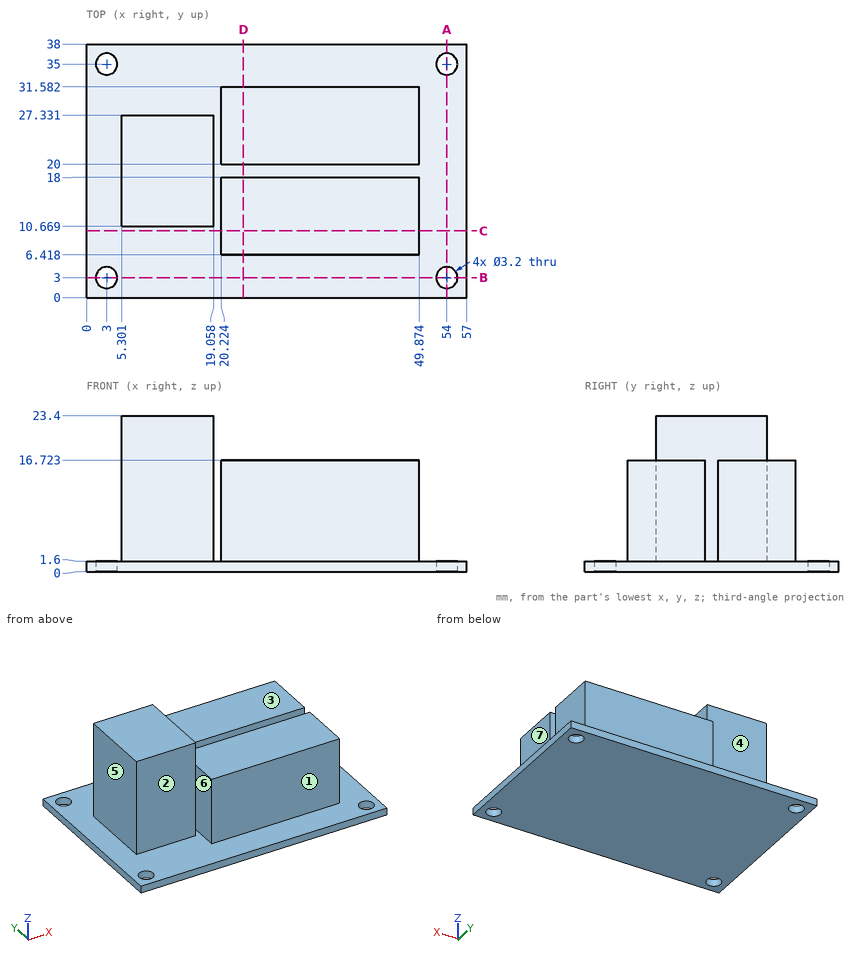
For this review, use the dimensioned drawing (mm, ordinates from the lowest corner) and the shaded views. A direction names the side the tool comes from. Round coordinates to 2 decimals unless told otherwise and drop trailing zeros. Loops run counter-clockwise (first coordinate to the right, second up) from the corner with the lowest first, then second, coordinate; pieces in that order, holes last. Notation, with made-up numbers: M 63,-9 L 111,-9 A22 ccw 111,5 Z; hole C 28,-10.75 d10. An arc over 180 degrees is marked long. Answer as CSV lines item,"result".
1. We need section D-D (x = 23.5). Give the boundary of the cut face in (y, z).
Outcome:
outline,"M 0,0 L 38,0 L 38,1.6 L 31.58,1.6 L 31.58,16.72 L 20,16.72 L 20,1.6 L 18,1.6 L 18,16.72 L 6.42,16.72 L 6.42,1.6 L 0,1.6 Z"
2. Insertion check: pin 1 Ø8.5 at (y, z) = (20.5, 9) entering from -X; pin 2 Ø3 at (x, z) = (22.5, 20) entering from +Y; pin 3 Ø3.5 at (y, z) = (13.5, 10) entering from +X; pin 4 Ø12 at (x, z) = (30, 12) entering from +Y. Each pin has a flat end and moves straight along its axis. Give the tip position at first contact, or say it passes through.
Outcome:
pin 1,"stops at x = 5.3"
pin 2,"passes through"
pin 3,"stops at x = 49.87"
pin 4,"stops at y = 31.58"
3. For the marked faces 1, 2 and 3, list the 3-axis set-ups (+Z, -Z, +X, -X, +Y, -Y) from which the entire face can be reached by the end or side of a thin tool; tool diameter is ignored.
Outcome:
face 1,"+Z, +X, -X, -Y"
face 2,"+Z, -X, -Y"
face 3,"+Z, +X, +Y, -Y"
4. We need section A-A (x = 54). Give the boundary of the cut face in (y, z).
Outcome:
outline,"M 0,0 L 1.4,0 L 1.4,1.6 L 0,1.6 Z; M 4.6,0 L 33.4,0 L 33.4,1.6 L 4.6,1.6 Z; M 36.6,0 L 38,0 L 38,1.6 L 36.6,1.6 Z"
5. We need section B-B (y = 3). Give the boundary of the cut face in (x, z).
Outcome:
outline,"M 0,0 L 1.4,0 L 1.4,1.6 L 0,1.6 Z; M 4.6,0 L 52.4,0 L 52.4,1.6 L 4.6,1.6 Z; M 55.6,0 L 57,0 L 57,1.6 L 55.6,1.6 Z"
6. To check wall thickness, follow L1, parallel to Y at x = 3, z = 0.35; L2, parallel to X at y = 14, z = 16.5; L3, parallel to Z at x = 39.5, y = 8. State the ranges of each line that lie inside material, in increasing order. Write a range as [from, to].
Outcome:
L1,"y = [0, 1.4], [4.6, 33.4], [36.6, 38]"
L2,"x = [5.3, 19.06], [20.22, 49.87]"
L3,"z = [0, 16.72]"
7. We need section C-C (y = 10). Give the boundary of the cut face in (x, z).
Outcome:
outline,"M 0,0 L 57,0 L 57,1.6 L 49.87,1.6 L 49.87,16.72 L 20.22,16.72 L 20.22,1.6 L 0,1.6 Z"
8. Draft analysis for pull direction X (two halves, no side actions). For the marked faces 4, 5, 6 and 7, state which applies: pulls with the +X half, pulls with the -X half, needs draft (parallel to the pull), parting line crosses it, or undercut.
Outcome:
face 4,"needs draft"
face 5,"pulls with the -X half"
face 6,"undercut"
face 7,"pulls with the +X half"
